Autodesk Inventor part; units mm, degrees
ref_plane "YZ Plane" through (0, 0, 0) normal (1, 0, 0) x (0, 1, 0)
ref_plane "XZ Plane" through (0, 0, 0) normal (0, 1, 0) x (-1, 0, 0)
ref_plane "XY Plane" through (0, 0, 0) normal (0, 0, 1) x (1, 0, 0)
sketch "Base" plane through (0, 0, 0) normal (0, 0, 1) x (1, 0, 0)
  line L0 (-1.9365, 3.5) -> (1.9365, 3.5)
  arc A0 (3.5, 1.9365) -> (1.9365, 3.5) centre (0, 0) ccw
  line L1 (3.5, 1.9365) -> (3.5, -1.9365)
  arc A1 (-1.9365, 3.5) -> (3.5, -1.9365) centre (0, 0) ccw
  circle A2 centre (0, 15.5) radius 1.65 construction
  circle A3 centre (13.4234, 7.75) radius 1.65 construction
  circle A4 centre (13.4234, -7.75) radius 1.65 construction
  circle A5 centre (0, -15.5) radius 1.65 construction
  circle A6 centre (-13.4234, -7.75) radius 1.65 construction
  circle A7 centre (-13.4234, 7.75) radius 1.65 construction
  circle A8 centre (0, 0) radius 39.5
  circle A9 centre (0, 15.5) radius 1.7
  circle A10 centre (-13.4234, 7.75) radius 1.7
  circle A11 centre (-13.4234, -7.75) radius 1.7
  circle A12 centre (0, -15.5) radius 1.7
  circle A13 centre (13.4234, -7.75) radius 1.7
  circle A14 centre (13.4234, 7.75) radius 1.7
  circle A15 centre (0, 0) radius 30
  point P0 (0, 0)
  dimension "d1" = 3.4
extrude "Plate1" add sketch "Base" along normal blind 5 contours A15
equation "\"d0\" = Thickness"
equation "\"BendRadius\" = Thickness"
equation "\"BendReliefWidth\" = Thickness"
equation "\"BendReliefDepth\" = 0.5 * Thickness"
equation "\"TransitionRadius\" = BendRadius"
equation "\"JacobiRadiusSize\" = BendRadius"
equation "\"GapSize\" = Thickness"
properties part number "NeckInnerFlange"
Here's how the part is built. I have some questions about the finished solid (model axes, mm). A direction names the side the tool comes from. Give positions to 0.01 mm unless a question says otherwise; leave off trailing zeros. Loops run counter-clockwise (first coordinate to the right, second up) from the corner with the lowest first, then second, coordinate; pieces in that order, holes last. Notation, with made-up numbers: (-27, 85) -> (-5, 85) arc R22 ccw to (-5, 121) -> close; hole circle Ø8 at (73, 33). An arc over 180 degrees is marked (long way). Answer as a JSON object with one key per item and string values. Group by question number.
Item 1: Will these pins go through, and if not, where does the flat tip stop? pin 1 (4 mm diameter, centred on x = 0, y = 15.5, fed in from +Z); pin 2 (1.2 mm diameter, centred on x = 0, z = 2.5, fed in from -Y).
Item 2: On a 3-axis mill with a long thin cutter (end or side, diameter ignored), from which of +Z, -Z, +X, -X, +Y, -Y can I reach the whole of each face in a straight line? I mean faces 1 (the flat face through (0, -6, 5)), 2 (the flat face through (3.5, 0, 2)). Say none if no direction works.
Item 3: Imagine slicing it at D-D on y = -7.75. Write out the boundary of the cut face in (x, z), then the cut area to 3 significant figures.
Item 4: Imagine slicing it at A-A on y = 0. Write out the boundary of the cut face in (x, z), then the cut area to 4 significant figures.
Item 5: Imagine slicing it at B-B on x = 0. Write out the boundary of the cut face in (y, z), then the cut area to 4 significant figures.
Item 6: I need wall thicknesses on L1, parallel to Y at x = 0, z = 3.25; L2, parallel to Y at x = -14, z = 2.4; L3, parallel to Y at x = 1, z = 3.8. Which ranges of each line are inside material? Lowest first, please.
Item 7: Imagine slicing it at C-C on z = 2.65. Write out the boundary of the cut face in (x, y), then the cut area to 3 significant figures.
Item 8: Thinking about a two-plate mould opening in X: for faces 3 (the flat face through (0, 3.5, 2)), 4 (the cylindrical face through (15.045, -8.261, 2.465)), 5 (the cylindrical face through (-29.97, -1.32, 2.46)), 6 (the flat face through (0, -6, 0)), which applies, pulls with the +X half, pulls with the -X half, needs draft (parallel to the pull), parting line crosses it, or undercut?
Answer list:
{
 "1": {"pin 1": "stops at z = 5", "pin 2": "stops at y = -30"},
 "2": {"face 1": "+Z, +X, -X, +Y, -Y", "face 2": "+Z, -Z"},
 "3": {"outline": "(-28.98, 0) -> (-15.12, 0) -> (-15.12, 5) -> (-28.98, 5) -> close; (-11.72, 0) -> (11.72, 0) -> (11.72, 5) -> (-11.72, 5) -> close; (15.12, 0) -> (28.98, 0) -> (28.98, 5) -> (15.12, 5) -> close", "area": "256 mm2"},
 "4": {"outline": "(-30, 0) -> (-4, 0) -> (-4, 5) -> (-30, 5) -> close; (3.5, 0) -> (30, 0) -> (30, 5) -> (3.5, 5) -> close", "area": "262.5 mm2"},
 "5": {"outline": "(-30, 0) -> (-17.2, 0) -> (-17.2, 5) -> (-30, 5) -> close; (-13.8, 0) -> (-4, 0) -> (-4, 5) -> (-13.8, 5) -> close; (3.5, 0) -> (13.8, 0) -> (13.8, 5) -> (3.5, 5) -> close; (17.2, 0) -> (30, 0) -> (30, 5) -> (17.2, 5) -> close", "area": "228.5 mm2"},
 "6": {"L1": "y = -30 to -17.2, -13.8 to -4, 3.5 to 13.8, 17.2 to 30", "L2": "y = -26.53 to -9.35, -6.15 to 6.15, 9.35 to 26.53", "L3": "y = -29.98 to -16.87, -14.13 to -3.87, 3.5 to 14.13, 16.87 to 29.98"},
 "7": {"outline": "circle Ø60 at (0, 0); hole circle Ø3.4 at (-13.42, -7.75); hole circle Ø3.4 at (-13.42, 7.75); hole (-1.94, 3.5) arc R4 ccw (long way) to (3.5, -1.94) -> (3.5, 1.94) arc R4 ccw to (1.94, 3.5) -> close; hole circle Ø3.4 at (0, -15.5); hole circle Ø3.4 at (0, 15.5); hole circle Ø3.4 at (13.42, -7.75); hole circle Ø3.4 at (13.42, 7.75)", "area": "2,730 mm2"},
 "8": {"face 3": "undercut", "face 4": "undercut", "face 5": "parting line crosses it", "face 6": "needs draft"}
}
